Verification items for the finished model (mm, model axes). A direction names the side the tool comes from. Coordinates: 2 decimals unless noted, no trailing zeros.
Q1. Set-up check for faces 1 (the flat face through (-76.2, -55, -15)), 2 (the flat face through (-3, 2, 0)): record each of +Z, -Z, +X, -X, +Y, -Y from which the full face is reachable in a straight line by a thin tool's end or side.
Q2. Cross-section at A-A, the plane z = -5.5. Count the separate pieces of the cut face and the enclosed holes in it, and give its area (3 significant figures).
Q3. Depth check by flat-ended pin: P1, Ø1, axis at y = -51, z = -25, coming from the +X side; P2, Ø15.5, axis at x = 3, z = -9, coming from the -Y side; P3, Ø9.5, axis at y = -52, z = -9.5, coming from the -X side; P4, Ø14.5, axis at x = -175, y = -30, coming from the +Z side. Enter the tip coordinate at first touch or a pass-through.
Q4. Draft check along Y on faces 3 (the flat face through (-3, 2, -31.055)), 4 (the cylindrical face through (166, -30, -15)). Enter one of: pulls with the +Y half, pulls with the -Y half, needs draft (parallel to the pull), parting line crosses it, or undercut.
Q5. Thickness scan on line 1 (Y direction, x = -1.5, z = -21); line 2 (Y direction, x = 34.5, z = -28.5); line 3 (Y direction, x = -175, z = -16). Record the ranges inside material, lowest first.
from build123d import *

# Parameters (mm, degrees)
SKETCH1_RX          = 240
SKETCH1_RY          = 110
BOSS_EXTRUDE1_DEPTH = 31.055
SKETCH10_W          = 254.8
SKETCH10_H          = 50.8
CUT_EXTRUDE5_DEPTH  = 266.827788286
SKETCH13_W          = 152.4
SKETCH13_H          = 78.9
CUT_EXTRUDE7_DEPTH  = 266.827788286
SKETCH12_R          = 9
CUT_EXTRUDE8_DEPTH  = 266.827788286


with BuildPart() as part:
    # Sketch1 → Boss-Extrude1 (new body)
    with BuildSketch(Plane.XY):
        with Locations((0, 0)):
            Ellipse(SKETCH1_RX, SKETCH1_RY)
    extrude(amount=-BOSS_EXTRUDE1_DEPTH)

    # Sketch10 → Cut-Extrude5 (cut, through all)
    with BuildSketch(Plane.XY):
        with Locations((0, 53.5)):
            Rectangle(SKETCH10_W, SKETCH10_H)
    extrude(amount=-CUT_EXTRUDE5_DEPTH, mode=Mode.SUBTRACT)

    # Sketch13 → Cut-Extrude7 (cut, through all)
    with BuildSketch(Plane.XY):
        with Locations((0, -54.45)):
            Rectangle(SKETCH13_W, SKETCH13_H)
    extrude(amount=-CUT_EXTRUDE7_DEPTH, mode=Mode.SUBTRACT)

    # Sketch12 → Cut-Extrude8 (cut, through all)
    with BuildSketch(Plane.XY):
        with Locations((175, -30)):
            Circle(SKETCH12_R)
        with Locations(Location((-175, -30, 0), (0, 0, 180))):
            Circle(SKETCH12_R)
    extrude(amount=-CUT_EXTRUDE8_DEPTH, mode=Mode.SUBTRACT)


solid = part.part
Check values:
1. face 1: +Z, -Z
1. face 2: +Z, +X, -X, +Y, -Y
2. separate pieces: 1
2. enclosed holes: 4
2. area: 57,500 mm2
3. P1: stops at x = 213.21
3. P2: stops at y = -110
3. P3: stops at x = -216.73
3. P4: passes through
4. face 3: needs draft
4. face 4: undercut
5. line 1: y = -110 to -93.9, -15 to 28.1, 78.9 to 110
5. line 2: y = -108.86 to -93.9, -15 to 28.1, 78.9 to 108.86
5. line 3: y = -75.28 to -39, -21 to 75.28
